from build123d import *

# Parameters (mm, degrees)
BOSS_EXTRUDE1_DEPTH = 260
SKETCH3_R           = 2.5
CUT_EXTRUDE1_DEPTH  = 261.384331326
CIRPATTERN1_COUNT   = 4


with BuildPart() as part:
    # Sketch2 → Boss-Extrude1 (new body)
    with BuildSketch(Plane(origin=(0, 0, 0), x_dir=(1, 0, 0), z_dir=(0, 1, 0))):
        with BuildLine():
            Line((-10, -8.5), (-10, 8.5))
            ThreePointArc((-10, 8.5), (-9.560660172, 9.560660172), (-8.5, 10))
            Line((-8.5, 10), (8.5, 10))
            ThreePointArc((8.5, 10), (9.560660172, 9.560660172), (10, 8.5))
            Line((10, 8.5), (10, -8.5))
            ThreePointArc((10, -8.5), (9.560660172, -9.560660172), (8.5, -10))
            Line((8.5, -10), (-8.5, -10))
            ThreePointArc((-8.5, -10), (-9.560660172, -9.560660172), (-10, -8.5))
        make_face()
    extrude(amount=BOSS_EXTRUDE1_DEPTH)

    # Sketch3 → Cut-Extrude1 (cut, through all)
    with BuildSketch(Plane(origin=(0, 260, 0), x_dir=(1, 0, 0), z_dir=(0, 1, 0))):
        with BuildLine():
            Line((-6.348528137, -5.5), (-4.2, -3.351471863))
            Line((-4.2, -3.351471863), (-4.2, 3.351471863))
            Line((-4.2, 3.351471863), (-6.348528137, 5.5))
            Line((-6.348528137, 5.5), (-8.5, 5.5))
            Line((-8.5, 5.5), (-8.5, 3.1))
            Line((-8.5, 3.1), (-9.3, 3.1))
            ThreePointArc((-9.3, 3.1), (-9.441421356, 3.158578644), (-9.5, 3.3))
            Line((-9.5, 3.3), (-9.5, 3.6))
            Line((-9.5, 3.6), (-9.8, 3.6))
            ThreePointArc((-9.8, 3.6), (-9.941421356, 3.658578644), (-10, 3.8))
            Line((-10, 3.8), (-10, -3.8))
            ThreePointArc((-10, -3.8), (-9.941421356, -3.658578644), (-9.8, -3.6))
            Line((-9.8, -3.6), (-9.5, -3.6))
            Line((-9.5, -3.6), (-9.5, -3.3))
            ThreePointArc((-9.5, -3.3), (-9.441421356, -3.158578644), (-9.3, -3.1))
            Line((-9.3, -3.1), (-8.5, -3.1))
            Line((-8.5, -3.1), (-8.5, -5.5))
            Line((-8.5, -5.5), (-6.348528137, -5.5))
        make_face()
        with Locations(Location((0, 0, 0), (0, 0, 270))):
            Circle(SKETCH3_R)
    cut_extrude1 = extrude(amount=-CUT_EXTRUDE1_DEPTH, mode=Mode.SUBTRACT)

    # CirPattern1: Cut-Extrude1 ×4 about axis
    cirpattern1_axis = Axis((0, 0, 0), (0, 1, 0))
    for i in range(1, CIRPATTERN1_COUNT):
        add(cut_extrude1.rotate(cirpattern1_axis, i * 360 / CIRPATTERN1_COUNT), mode=Mode.SUBTRACT)


solid = part.part
Read the model definition and answer for the solid it produces. Units are mm, in the model's axes. Coordinates: 2 decimals unless noted, no trailing zeros. Write each loop counter-clockwise with the first axis right and the second up, starting at its lowest first coordinate (ties: lowest second). Pieces come first, ordered by that corner, then holes. Notation, with made-up numbers: M 58,45.25 L 106,45.25 A16 ccw 106,60.25 Z; hole C 6.5,41.25 d10. An arc over 180 degrees is marked long. Use a Markdown table: item, result.
Q1. Straight lines are drawn through the part: L1, parallel to X at y = 75.5, z = 7.75; L2, parallel to Z at x = 0, y = 74. For each, find the intervals that lie inside material, in ascending order. Write a range as [from, to].
Answer block:
| item | result |
|---|---|
| L1 | x = [-10, -5.5], [5.5, 10] |
| L2 | z = [-4.2, -2.5], [2.5, 4.2] |
Q2. The part is cut by section A-A, the plane z = 0. Write down the section's boundary in (x, y).
Answer block:
| item | result |
|---|---|
| outline | M -4.2,0 L -2.5,0 L -2.5,260 L -4.2,260 Z; M 2.5,0 L 4.2,0 L 4.2,260 L 2.5,260 Z |
Q3. Each of these flat-tipped pins is pushed along its axis until it touches: pin 1 Ø2 at (y, z) = (85.5, 1) entering from -X; pin 2 Ø5 at (y, z) = (95, 2) entering from +X; pin 3 Ø5.5 at (x, y) = (0.5, 65.5) entering from -Z. Where does it stop, or does it pass through?
Answer block:
| item | result |
|---|---|
| pin 1 | stops at x = -4.2 |
| pin 2 | stops at x = 10 |
| pin 3 | stops at z = -9.49 |
Q4. The part is cut by section B-B, the plane x = 0. Write down the section's boundary in (y, z), then the cut area to 3 significant figures.
Answer block:
| item | result |
|---|---|
| outline | M 0,-4.2 L 260,-4.2 L 260,-2.5 L 0,-2.5 Z; M 0,2.5 L 260,2.5 L 260,4.2 L 0,4.2 Z |
| area | 884 mm2 |
Q5. Determine the mould class of faces 1 (the face through (-6, 128, -10)), 2 (the face through (0, 132, -4.2)), 3 (the face through (-2.44, 131.82, -0.54)), 4 (the face through (-10, 128, 6)) for opening direction X: released by +X, released by -X, zero draft, split by the parting line, or undercut.
Answer block:
| item | result |
|---|---|
| face 1 | zero draft |
| face 2 | undercut |
| face 3 | undercut |
| face 4 | released by -X |
